from build123d import *

# Parameters (mm, degrees)
F0_W     = 110
F0_H     = 40
F1_DEPTH = 2
F2_W     = 100.4
F2_H     = 30.4
F3_DEPTH = 2.001
F4_R     = 4
F5_R     = 1.5


with BuildPart() as f1:
    # F0 (on Top) → F1 (new body)
    with BuildSketch(Plane.XY):
        Rectangle(F0_W, F0_H)
    extrude(amount=F1_DEPTH)

    # F2 (on face) → F3 (cut, through all)
    with BuildSketch(Plane.XY.offset(2)):
        Rectangle(F2_W, F2_H)
    extrude(amount=-F3_DEPTH, mode=Mode.SUBTRACT)

    # F4
    f4_edges = [f1.edges().sort_by_distance(p)[0] for p in [
        (-55, -20, 1),
        (-55, 20, 1),
        (55, -20, 1),
        (55, 20, 1),
    ]]
    fillet(f4_edges, radius=F4_R)

    # F5
    f5_edges = [f1.edges().sort_by_distance(p)[0] for p in [
        (-50.2, 15.2, 1),
        (50.2, 15.2, 1),
        (-50.2, -15.2, 1),
        (50.2, -15.2, 1),
    ]]
    fillet(f5_edges, radius=F5_R)


solid = f1.part
The listing builds one solid part. Answer for the finished solid, in the listing's coordinates (mm). A direction names the side the tool comes from. Coordinates: 2 decimals unless noted, no trailing zeros. Write each loop counter-clockwise with the first axis right and the second up, starting at its lowest first coordinate (ties: lowest second). Pieces come first, ordered by that corner, then holes. Notation, with made-up numbers: (-9.75, -24) -> (20.25, -24) arc R16 ccw to (20.25, -17) -> close; hole circle Ø1 at (47.25, 21). An arc over 180 degrees is marked (long way). One line per question, with ' | ' between items.
1. Given pin 1 Ø12 at (x, y) = (22.5, 6.5) entering from -Z, flat-ended and moving along its own axis, determine where the tip first touches the part or whether it passes through.
Verdict:
pin 1: passes through
2. Section C-C (x = 38.5) is taken. Determine the outline of the cut face in (y, z).
Verdict:
outline: (-20, 0) -> (-15.2, 0) -> (-15.2, 2) -> (-20, 2) -> close; (15.2, 0) -> (20, 0) -> (20, 2) -> (15.2, 2) -> close
3. For a pull along X with two mould halves and no side action, classify faces 1 (the flat face through (50.2, 0, 1)), 2 (the flat face through (55, 0, 1)), 3 (the flat face through (-1, -15.2, 1)), 4 (the cylindrical face through (-53.859, 18.797, 1.014)) as released by +X, released by -X, zero draft, split by the parting line, or undercut.
Verdict:
face 1: undercut | face 2: released by +X | face 3: undercut | face 4: released by -X
4. Section B-B (z = 1.35) is taken. Determine the outline of the cut face in (x, y), and give its area (3 significant figures).
Verdict:
outline: (-55, -16) arc R4 ccw to (-51, -20) -> (51, -20) arc R4 ccw to (55, -16) -> (55, 16) arc R4 ccw to (51, 20) -> (-51, 20) arc R4 ccw to (-55, 16) -> close; hole (-50.2, -13.7) arc R1.5 ccw to (-48.7, -15.2) -> (48.7, -15.2) arc R1.5 ccw to (50.2, -13.7) -> (50.2, 13.7) arc R1.5 ccw to (48.7, 15.2) -> (-48.7, 15.2) arc R1.5 ccw to (-50.2, 13.7) -> close | area: 1,340 mm^2
5. Section A-A (y = -6.5) is taken. Determine the outline of the cut face in (x, z).
Verdict:
outline: (-55, 0) -> (-50.2, 0) -> (-50.2, 2) -> (-55, 2) -> close; (50.2, 0) -> (55, 0) -> (55, 2) -> (50.2, 2) -> close
6. Which of the six approach directions +Z, -Z, +X, -X, +Y, -Y give full straight-line access (tool end or side, diameter ignored) to faces 5 (the flat face through (-50.2, 0, 1)), 6 (the flat face through (4, -16, 2))?
Verdict:
face 5: +Z, -Z | face 6: +Z, +X, -X, +Y, -Y
7. Straight lines are drawn through the part: line 1 (X direction, y = -1, z = 1.7); line 2 (Y direction, x = -32, z = 1.85); line 3 (Y direction, x = 50, z = 0.6). For each, find the intervals that lie inside material, in ascending order.
Verdict:
line 1: x = -55 to -50.2, 50.2 to 55 | line 2: y = -20 to -15.2, 15.2 to 20 | line 3: y = -20 to -14.45, 14.45 to 20
